Autodesk Inventor part; units mm, degrees
ref_plane "YZ Plane" through (0, 0, 0) normal (1, 0, 0) x (0, 1, 0)
ref_plane "XZ Plane" through (0, 0, 0) normal (0, 1, 0) x (-1, 0, 0)
ref_plane "XY Plane" through (0, 0, 0) normal (0, 0, 1) x (1, 0, 0)
sketch "Skizze1" plane through (0, 0, 0) normal (0, 0, 1) x (1, 0, 0)
  line L0 (-7, 0) -> (7, 0)
  line L1 (0, -30) -> (0, 5)
  line L2 (5, -20) -> (-5, -20)
  line L3 (-5, -20) -> (-5, 0)
  line L4 (-5, 0) -> (5, 0)
  line L5 (5, 0) -> (5, -20)
  line L6 (5, -20) -> (-5, 0) construction
  line L7 (-5, -20) -> (5, 0) construction
  arc A0 (-5, -20) -> (5, -20) centre (0, -20) ccw
  point P0 (0, 0)
  point P1 (0, -10)
  dimension "d0" = 10
  dimension "d1" = 20
extrude "Extrusion1" add sketch "Skizze1" along normal blind 3
sketch "Skizze2" plane through (5, -20, 0) normal (1, 0, 0) x (0, 0, -1)
  line L0 (0, 0) -> (0, 20)
  line L1 (0, 20) -> (-3, 20)
  line L2 (-3, 0) -> (-3, 20)
  line L3 (0, 0) -> (-3, 0)
  line L4 (-3, 0) -> (-3, 20)
  line L5 (-3, 9.5) -> (-2.1, 9.5)
  line L6 (-2.1, 9.5) -> (-2.1, 19.5)
  line L7 (-2.1, 19.5) -> (-3, 19.5)
  line L8 (-3, 19.5) -> (-3, 9.5)
  point P0 (0, 20)
  point P1 (-2.55, 19.5)
  point P2 (-3, 19.5)
  dimension "d4" = 0.9
  dimension "d5" = 0.5
  dimension "d6" = 10
extrude "Extrusion2" cut sketch "Skizze2" against normal through all contours L2 L7 L6 L5
sketch "Skizze4" plane through (0, 0, 0) normal (0, 0, -1) x (-1, 0, 0)
  arc A0 (-5, -20) -> (5, -20) centre (0, -20) ccw
  line L0 (5, 0) -> (5, -20)
  line L1 (-5, 0) -> (5, 0)
  line L2 (-5, -20) -> (-5, 0)
  line L3 (0, -32.4) -> (0, 5.4)
  line L4 (7, 0) -> (-7, 0)
  point P0 (0, 0)
  point P1 (0, -15)
  dimension "d9" = 5
hole "Bohrung1" at (0, -15, 0) direction (0, 0, 1) diameter 4.5 end through all countersink diameter 9.2 countersink angle 90
sketch "Skizze5" plane through (0, 0, 0) normal (0, 0, -1) x (-1, 0, 0)
  line L0 (0, -30) -> (0, 5)
  line L1 (7, 0) -> (-7, 0)
  circle A0 centre (0, -15) radius 4.6
  point P0 (0, 0)
  point P1 (0, -22)
  dimension "d17" = 7
hole "Bohrung2" at (0, -22, 0) direction (0, 0, 1) diameter 3 end through all
properties part number "24_0497_007"
Geometry: final body of the model. Coordinates: model frame, mm. A direction names the side the tool comes from. Coordinates: 2 decimals unless noted, no trailing zeros. Order: outer loops, then holes, each group sorted by start corner. A loop starts at its lowest first (then second) coordinate and runs counter-clockwise, first axis right, second up. Notation, with made-up numbers: M -2,-20.75 L 45,-20.75 A11 cw 45,-4.75 Z; hole C 45,8.5 d2. An arc over 180 degrees is marked long. Answer in a Markdown table with one row per item. Add a question column.
Q1. Section query A-A on y = -15. Return the cut outline in (x, z), and give its area (3 significant figures).
Q2. Line query: L1, parallel to Y at x = 0, z = 2.75; L2, parallel to X at y = -14.5, z = 2.3 (3 decimals); L3, parallel to Y at x = 0, z = 1.45. Output: solid intervals per line, ascending.
Q3. Contact query for a flat-ended pin moving along its axis: P1, Ø1.8, axis at x = 0, y = -22, coming from the +Z side. Output: stop coordinate, or through.
Q4. Mould query, pull axis Y, two halves, no side actions, for faces 3 (the cylindrical face through (-0.676, -12.854, 2.68)), 4 (the flat face through (0, -18, 3)), 5 (the cylindrical face through (0, -25, 1)), 6 (the flat face through (0, 0, 1)). Classes: released by +Y, released by -Y, zero draft, split by the parting line, or undercut.
Q5. Section query C-C on x = 0. Return the cut outline in (y, z), and give its area (3 significant figures).
Q6. Section query D-D on y = -10. Return the cut outline in (x, z), and give its area (3 significant figures).
Q7. Reachability of faces 1 (the flat face through (0, -6, 2.1)), 2 (the cylindrical face through (-0.07, -23.5, 1.52)) from +Z, -Z, +X, -X, +Y, -Y: full face, straight path, thin tool, end or side. Return the list, or none.
Q8. Section query B-B on z = 1.3. Return the cut outline in (x, y).
Completed:
| question | item | result |
|---|---|---|
| 1 | outline | M -5,0 L -4.6,0 L -2.25,2.35 L -2.25,3 L -5,3 Z; M 2.25,2.35 L 4.6,0 L 5,0 L 5,3 L 2.25,3 Z |
| 1 | area | 11.0 mm2 |
| 2 | L1 | y = -25 to -23.5, -20.5 to -17.25, -12.75 to -10.5, -0.5 to 0 |
| 2 | L2 | x = -5 to -2.245, 2.245 to 5 |
| 2 | L3 | y = -25 to -23.5, -20.5 to -18.15, -11.85 to 0 |
| 3 | P1 | passes through |
| 4 | face 3 | undercut |
| 4 | face 4 | zero draft |
| 4 | face 5 | released by -Y |
| 4 | face 6 | released by +Y |
| 5 | outline | M -25,0 L -23.5,0 L -23.5,3 L -25,3 Z; M -20.5,0 L -19.6,0 L -17.25,2.35 L -17.25,3 L -20.5,3 Z; M -12.75,2.35 L -10.4,0 L 0,0 L 0,3 L -0.5,3 L -0.5,2.1 L -10.5,2.1 L -10.5,3 L -12.75,3 Z |
| 5 | area | 38.0 mm2 |
| 6 | outline | M -5,0 L 5,0 L 5,2.1 L -5,2.1 Z |
| 6 | area | 21.0 mm2 |
| 7 | face 1 | +Z, +X, -X |
| 7 | face 2 | +Z, -Z |
| 8 | outline | M -5,-20 A5 ccw 5,-20 L 5,0 L -5,0 Z; hole C 0,-15 d6.6; hole C 0,-22 d3 |
